The drawing under review shows one solid part. Ordinate dimensions are in mm from its lowest x, y, z. A direction names the side the tool comes from. Coordinates: 2 decimals unless noted, no trailing zeros. Order: outer loops, then holes, each group sorted by start corner. A loop starts at its lowest first (then second) coordinate and runs counter-clockwise, first axis right, second up. Notation, with made-up numbers: (14, 65.5) - (68, 65.5) arc R19 ccw to (68, 71.5) - close; hole circle Ø1 at (81.5, 5.5). An arc over 180 degrees is marked (long way). Answer in a Markdown table with one row per item.
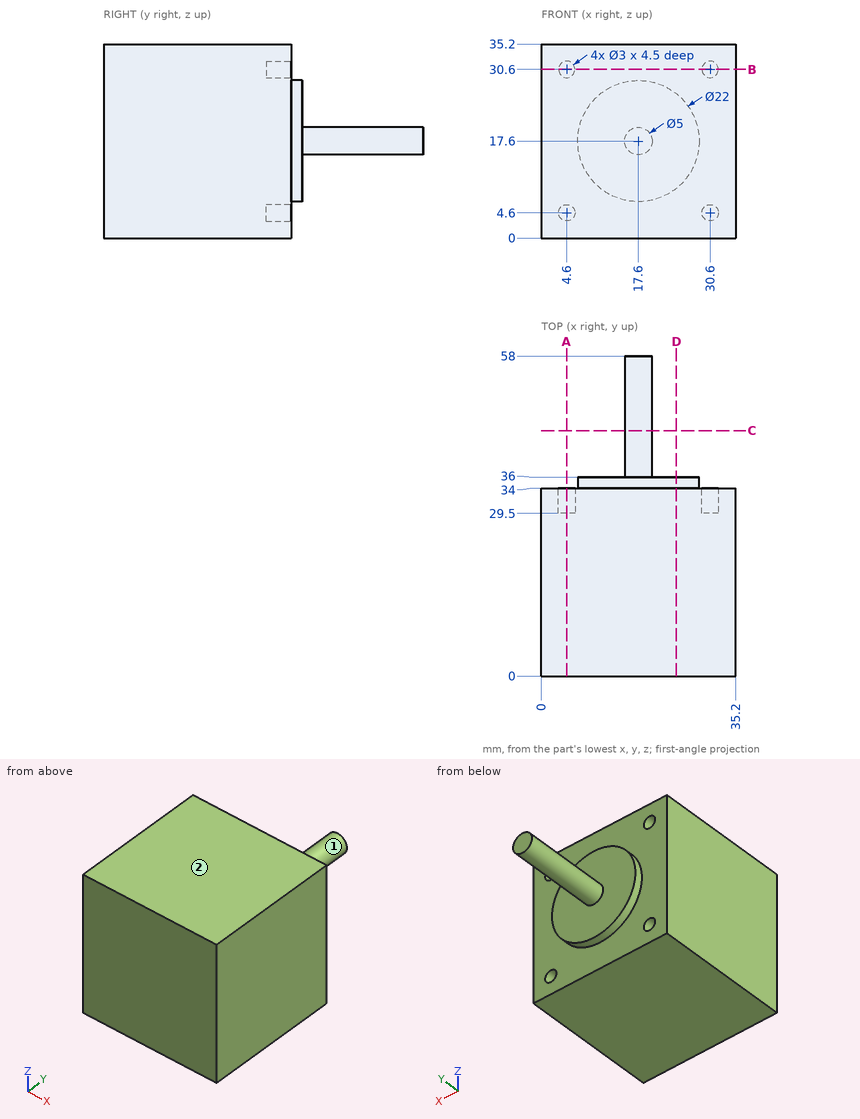
Item 1: To check wall thickness, follow line 1 (Z direction, x = 30.6, y = 32.7); line 2 (X direction, y = 30, z = 30); line 3 (Y direction, x = 21.5, z = 19.5). State the ranges of each line that lie inside material, in increasing order. Write a range as from..to.
Check values:
| item | result |
|---|---|
| line 1 | 0..3.1, 6.1..29.1, 32.1..35.2 |
| line 2 | 0..3.23, 5.97..29.23, 31.97..35.2 |
| line 3 | 0..36 |
Item 2: We need section D-D, the plane x = 24.5. Write out the cut boundary in (y, z).
Check values:
| item | result |
|---|---|
| outline | (0, 0) - (34, 0) - (34, 9.03) - (36, 9.03) - (36, 26.17) - (34, 26.17) - (34, 35.2) - (0, 35.2) - close |
Item 3: We need section B-B, the plane z = 30.6. Write out the cut boundary in (x, y).
Check values:
| item | result |
|---|---|
| outline | (0, 0) - (35.2, 0) - (35.2, 34) - (32.1, 34) - (32.1, 29.5) - (29.1, 29.5) - (29.1, 34) - (6.1, 34) - (6.1, 29.5) - (3.1, 29.5) - (3.1, 34) - (0, 34) - close |
Item 4: We need section C-C, the plane y = 44.5. Write out the cut boundary in (x, z).
Check values:
| item | result |
|---|---|
| outline | circle Ø5 at (17.6, 17.6) |
Item 5: Clearance check with flat-ended pins moving along their axes: pin 1 Ø4 at (x, z) = (28.5, 26.5) entering from +Y; pin 2 Ø1.8 at (x, z) = (30.6, 30.6) entering from +Y. State where each tip first meets the part, or that it passes through.
Check values:
| item | result |
|---|---|
| pin 1 | y = 34 |
| pin 2 | y = 29.5 |
Item 6: We need section A-A, the plane x = 4.6. Write out the cut boundary in (y, z), then the cut area to 3 significant figures.
Check values:
| item | result |
|---|---|
| outline | (0, 0) - (34, 0) - (34, 3.1) - (29.5, 3.1) - (29.5, 6.1) - (34, 6.1) - (34, 29.1) - (29.5, 29.1) - (29.5, 32.1) - (34, 32.1) - (34, 35.2) - (0, 35.2) - close |
| area | 1,170 mm^2 |
Item 7: Tool access review of the marked faces 1 and 2: name each direction out of +Z, -Z, +X, -X, +Y, -Y from which nothing blocks a thin tool from reaching the whole face with its end or side.
Check values:
| item | result |
|---|---|
| face 1 | +Y |
| face 2 | +Z, +X, -X, +Y, -Y |
